Here's the drawing with two shaded views (mm, measured from the low corner). I have some questions. Round coordinates to 2 decimals unless told otherwise and drop trailing zeros. Order: outer loops, then holes, each group sorted by start corner. A loop starts at its lowest first (then second) coordinate and runs counter-clockwise, first axis right, second up. Notation, with made-up numbers: (39, 70.25) -> (78, 70.25) arc R16 cw to (78, 75.25) -> close; hole circle Ø9 at (47.5, -8.75). An arc over 180 degrees is marked (long way). Use a Markdown table: item, result. Add a question column.
Q1. I'm going to push flat-ended pins straight in: pin 1 Ø1 at (x, z) = (11.5, 88) entering from -Y; pin 2 Ø3 at (x, z) = (70.5, 176.5) entering from +Y; pin 3 Ø1.5 at (y, z) = (39, 48.5) entering from -X. Where does each tip first touch, or does it pass through?
Q2. If we section it at D-D on z = 146: List the corners of the cut face in (x, y) for me, plus the area to 3 significant figures.
Q3. I need wall thicknesses on line 1 along Z through (x, y) = (83, 16.5); line 2 along Y through (x, z) = (11.5, 238); line 3 along Y through (x, z) = (62, 72). Which ranges of each line are inside material? Lowest first, please. Write a range as [from, to].
Q4. If we section it at B-B on y = 50: List the corners of the cut face in (x, z) for me, plus the area to 4 significant figures.
Q5. If we section it at A-A on y = 6: List the corners of the cut face in (x, z) for me.
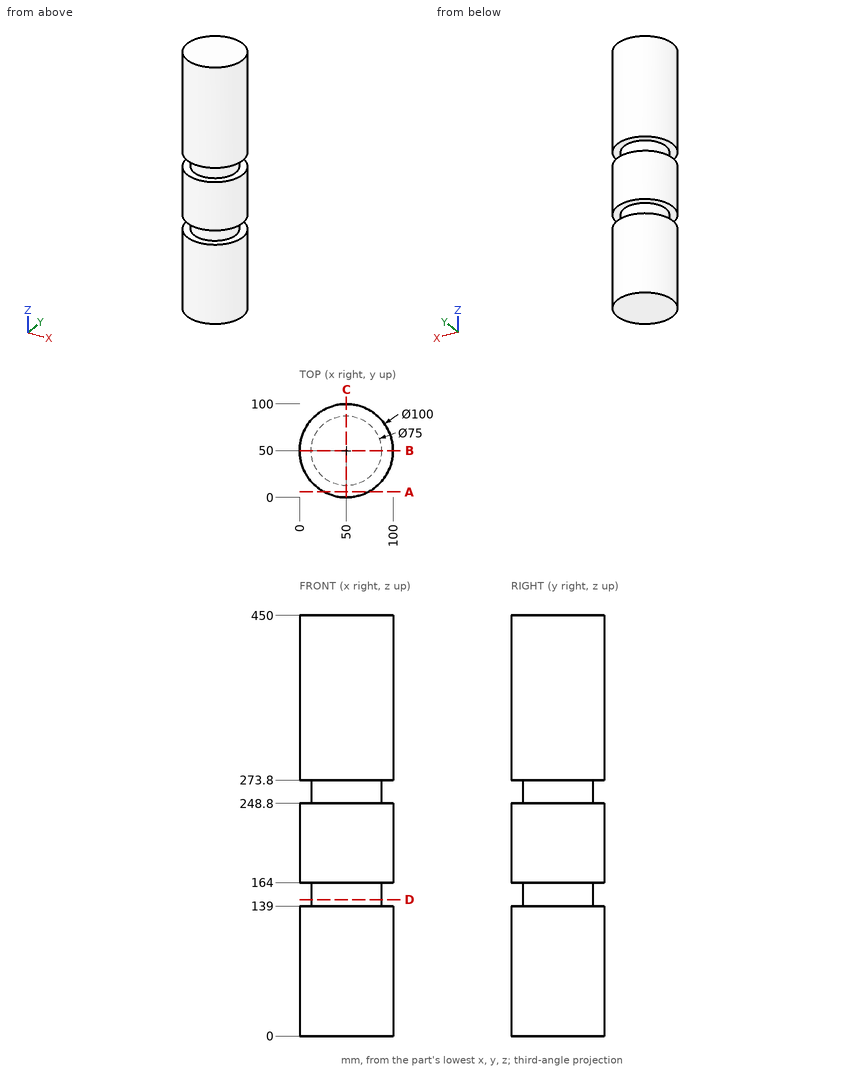
Answer below:
| question | item | result |
|---|---|---|
| 1 | pin 1 | y = 17.5 |
| 1 | pin 2 | y = 96.25 |
| 1 | pin 3 | x = 1.06 |
| 2 | outline | circle Ø75 at (50, 50) |
| 2 | area | 4,420 mm² |
| 3 | line 1 | [0, 139], [164, 248.8], [273.8, 450] |
| 3 | line 2 | [18.1, 81.9] |
| 3 | line 3 | [1.46, 98.54] |
| 4 | outline | (0, 0) -> (100, 0) -> (100, 139) -> (87.5, 139) -> (87.5, 164) -> (100, 164) -> (100, 248.8) -> (87.5, 248.8) -> (87.5, 273.8) -> (100, 273.8) -> (100, 450) -> (0, 450) -> (0, 273.8) -> (12.5, 273.8) -> (12.5, 248.8) -> (0, 248.8) -> (0, 164) -> (12.5, 164) -> (12.5, 139) -> (0, 139) -> close |
| 4 | area | 43,750 mm² |
| 5 | outline | (26.25, 0) -> (73.75, 0) -> (73.75, 139) -> (26.25, 139) -> close; (26.25, 164) -> (73.75, 164) -> (73.75, 248.8) -> (26.25, 248.8) -> close; (26.25, 273.8) -> (73.75, 273.8) -> (73.75, 450) -> (26.25, 450) -> close |
